from build123d import *

# Parameters (mm, degrees)
SKETCH1_W           = 240
SKETCH1_H           = 175
BOSS_EXTRUDE1_DEPTH = 5
SKETCH2_W           = 230
SKETCH2_H           = 165
CUT_EXTRUDE1_DEPTH  = 3
FILLET1_R           = 1
FILLET2_R           = 1
FILLET3_R           = 1


with BuildPart() as part:
    # Sketch1 → Boss-Extrude1 (new body)
    with BuildSketch(Plane.XY):
        with Locations((4.817749604, -19.687004754)):
            Rectangle(SKETCH1_W, SKETCH1_H)
    extrude(amount=BOSS_EXTRUDE1_DEPTH)

    # Sketch2 → Cut-Extrude1 (cut)
    with BuildSketch(Plane.XY.offset(5)):
        with Locations((4.817749604, -19.687004754)):
            Rectangle(SKETCH2_W, SKETCH2_H)
    extrude(amount=-CUT_EXTRUDE1_DEPTH, mode=Mode.SUBTRACT)

    # Fillet1
    fillet1_edges = [part.edges().sort_by_distance(p)[0] for p in [
        (4.817749604, -102.187004754, 2),
        (119.817749604, -102.187004754, 3.5),
        (-110.182250396, -102.187004754, 3.5),
        (4.817749604, 62.812995246, 5),
        (-110.182250396, -19.687004754, 5),
        (4.817749604, -102.187004754, 5),
        (119.817749604, -19.687004754, 5),
    ]]
    fillet(fillet1_edges, radius=FILLET1_R)

    # Fillet2
    fillet2_edges = [part.edges().sort_by_distance(p)[0] for p in [
        (124.817749604, -19.687004754, 5),
        (4.817749604, 67.812995246, 5),
        (-115.182250396, -19.687004754, 5),
        (4.817749604, -107.187004754, 5),
    ]]
    fillet(fillet2_edges, radius=FILLET2_R)

    # Fillet3
    # the kernel refuses this fillet: 1 mm, written as the material it adds along each edge
    with BuildSketch(Plane(origin=(118.817749604, -101.187004754, 3), x_dir=(0, 0, -1), z_dir=(1, 0, 0))) as fillet3_piece_1_section:
        Polygon((0, 0), (FILLET3_R, 0), (FILLET3_R, -FILLET3_R), (0, -FILLET3_R), align=None)
    fillet3_piece_1 = extrude(amount=FILLET3_R, mode=Mode.PRIVATE)
    fillet3_piece_1 = fillet3_piece_1 - Plane(origin=(118.817749604, -101.187004754, 3), x_dir=(0, 0.7071067811865475, 0.7071067811865475), z_dir=(1, 0, 0)) * Sphere(FILLET3_R, mode=Mode.PRIVATE)
    add(fillet3_piece_1)
    with BuildSketch(Plane(origin=(-109.182250396, -101.187004754, 3), x_dir=(0, 0, -1), z_dir=(-1, 0, 0))) as fillet3_piece_2_section:
        Polygon((0, 0), (FILLET3_R, 0), (FILLET3_R, FILLET3_R), (0, FILLET3_R), align=None)
    fillet3_piece_2 = extrude(amount=FILLET3_R, mode=Mode.PRIVATE)
    fillet3_piece_2 = fillet3_piece_2 - Plane(origin=(-109.182250396, -101.187004754, 3), x_dir=(0, 0.7071067811865475, 0.7071067811865475), z_dir=(-1, 0, 0)) * Sphere(FILLET3_R, mode=Mode.PRIVATE)
    add(fillet3_piece_2)
    with BuildSketch(Plane(origin=(122.317749604, 62.812995246, 2), x_dir=(0, 0, 1), z_dir=(-1, 0, 0))) as fillet3_piece_3:
        with BuildLine():
            CenterArc((FILLET3_R, -FILLET3_R), FILLET3_R, 90, 90)
            Line((0, -FILLET3_R), (0, 0))
            Line((0, 0), (FILLET3_R, 0))
        make_face()
    extrude(amount=235)
    with BuildSketch(Plane(origin=(-110.182250396, 65.312995246, 2), x_dir=(0, 0, 1), z_dir=(0, -1, 0)), Plane(origin=(119.817749604, -101.187004754, 2), x_dir=(0, 0, 1), z_dir=(0, 1, 0))) as fillet3_piece_4:
        with BuildLine():
            CenterArc((FILLET3_R, -FILLET3_R), FILLET3_R, 90, 90)
            Line((0, -FILLET3_R), (0, 0))
            Line((0, 0), (FILLET3_R, 0))
        make_face()
    extrude(amount=166.5)


solid = part.part
Work out the finished part from the listing and answer in its coordinate system (mm). Round coordinates to 2 decimals unless told otherwise and drop trailing zeros. Order: outer loops, then holes, each group sorted by start corner. A loop starts at its lowest first (then second) coordinate and runs counter-clockwise, first axis right, second up. Notation, with made-up numbers: M 14,-23 L 42,-23 A15 cw 42,-18 Z; hole C 38.5,5.5 d6. An arc over 180 degrees is marked long. One line per item, written item: value.
Q1. Straight lines are drawn through the part: line 1 (Y direction, x = 59.5, z = 3.7); line 2 (X direction, y = -75, z = 2.7); line 3 (X direction, y = 10.5, z = 3.3). For each, find the intervals that lie inside material, in ascending order.
Derived:
line 1: -107.19 to -102.19, 62.81 to 67.81
line 2: -115.18 to -110.14, 119.77 to 124.82
line 3: -115.18 to -110.18, 119.82 to 124.82
Q2. Find section B-B on x = -37. Write down the section's boundary in (y, z).
Derived:
outline: M -107.19,0 L 67.81,0 L 67.81,4 A1 ccw 66.81,5 L 63.81,5 A1 ccw 62.81,4 L 62.81,3 A1 cw 61.81,2 L -101.19,2 A1 cw -102.19,3 L -102.19,4 A1 ccw -103.19,5 L -106.19,5 A1 ccw -107.19,4 Z
Q3. Determine the mould class of faces 1 (the face through (3, -19, 2)), 2 (the face through (3, -18, 0)) for opening direction Y: released by +Y, released by -Y, zero draft, split by the parting line, or undercut.
Derived:
face 1: undercut
face 2: zero draft
Q4. A flat-ended cylindrical pin translates along its axis: pin 1 (1 mm diameter, centred on x = -56.5, y = -54.5, fed in from +Z). Find the tip coordinate at first contact, or state that the pin passes through.
Derived:
pin 1: z = 2
Q5. Find section A-A on y = 29. Write down the section's boundary in (x, z), then the cut area to 3 significant figures.
Derived:
outline: M -115.18,0 L 124.82,0 L 124.82,4 A1 ccw 123.82,5 L 120.82,5 A1 ccw 119.82,4 L 119.82,3 A1 cw 118.82,2 L -109.18,2 A1 cw -110.18,3 L -110.18,4 A1 ccw -111.18,5 L -114.18,5 A1 ccw -115.18,4 Z
area: 510 mm²
